from build123d import *

# Parameters (mm, degrees)
SKETCH1_W           = 310
SKETCH1_H           = 20
SKETCH1_W_2         = 20
SKETCH1_H_2         = 460
BOSS_EXTRUDE1_DEPTH = 62


with BuildPart() as part:
    # Sketch1 → Boss-Extrude1 (new body)
    with BuildSketch(Plane(origin=(0, 0, 0), x_dir=(1, 0, 0), z_dir=(0, 1, 0))):
        with Locations((175, 10)):
            Rectangle(SKETCH1_W, SKETCH1_H)
        with Locations((10, 230)):
            Rectangle(SKETCH1_W_2, SKETCH1_H_2)
        with Locations((175, 450)):
            Rectangle(SKETCH1_W, SKETCH1_H)
        Polygon((330, 20), (330, 0), (350, 0), (350, 460), (330, 460), (330, 440), align=None)
    extrude(amount=BOSS_EXTRUDE1_DEPTH)


solid = part.part
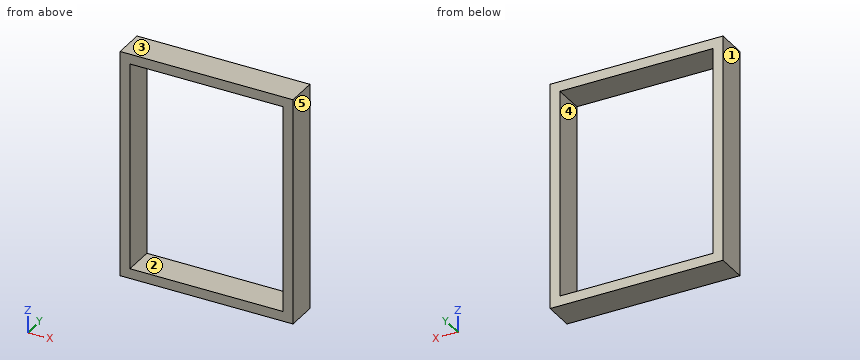
Design review of the part built by this model. Coordinates are the model's own, in mm. Face numbers are marked on the shaded views. A direction names the side the tool comes from. Give positions to 0.01 mm unless a question says otherwise; leave off trailing zeros. Order: outer loops, then holes, each group sorted by start corner. A loop starts at its lowest first (then second) coordinate and runs counter-clockwise, first axis right, second up. Notation, with made-up numbers: (30.25, -25) - (38.25, -25) arc R16 ccw to (38.25, -21) - close; hole circle Ø8 at (-32.75, 67). An arc over 180 degrees is marked (long way). Use CSV: the item, a comma, the result in double quotes. Start each with the question number.
Q1. Take a section at C-C (z = -302). State the section outline as (x, y) points, and give its area (3 significant figures).
Q2. Take a section at B-B (y = 12). State the section outline as (x, z) points, and give its area (3 significant figures).
Q3. Draft analysis for pull direction X (two halves, no side actions). For the marked faces 3, 4 and 5, state which applies: pulls with the +X half, pulls with the -X half, needs draft (parallel to the pull), parting line crosses it, or undercut.
Q4. For line 1 (Z direction, x = 134.5, y = 7); line 2 (X direction, y = 26, z = -146.5), list the stretches that pass through material, from the lowest coordinate up.
Q5. For P1, Ø3, axis at x = 150.5, y = 45.5, coming from the +Z side, flat-tipped, find the tip position at first contact; note if it passes through.
Q6. Machinability: for the marked faces 1 and 2, which of the approach directions +Z, -Z, +X, -X, +Y, -Y give a long, thin tool a straight path to every point of the face, cutting with its end or side? Answer none if there is none.
Q7. Take a section at A-A (x = 117). State the section outline as (y, z) points.
Calculated:
1,outline,"(0, 0) - (20, 0) - (20, 62) - (0, 62) - close; (330, 0) - (350, 0) - (350, 62) - (330, 62) - close"
1,area,"2,480 mm²"
2,outline,"(0, -460) - (350, -460) - (350, 0) - (0, 0) - close; hole (20, -440) - (330, -440) - (330, -20) - (20, -20) - close"
2,area,"30,800 mm²"
3,face 3,"needs draft"
3,face 4,"undercut"
3,face 5,"pulls with the +X half"
4,line 1,"z = -460 to -440, -20 to 0"
4,line 2,"x = 0 to 20, 330 to 350"
5,P1,"stops at z = 0"
6,face 1,"+Z, -Z, -X, +Y, -Y"
6,face 2,"+Y, -Y"
7,outline,"(0, -460) - (62, -460) - (62, -440) - (0, -440) - close; (0, -20) - (62, -20) - (62, 0) - (0, 0) - close"
